```python
from build123d import *

# Parameters (mm, degrees)
ESQUISSE_CYLINDRE_R = 4.5
CYLINDRE_DEPTH      = 29
EPAULEMENT_DEPTH    = 1.5
ESQUISSE_TROU_R     = 2
TROU_DEPTH          = 3.5
CHANFREIN1_SIZE     = 1


with BuildPart() as part:
    # Esquisse_cylindre → Cylindre (new body)
    with BuildSketch(Plane.XY):
        Circle(ESQUISSE_CYLINDRE_R)
    extrude(amount=-CYLINDRE_DEPTH)

    # Esquisse_épaulement → Epaulement (add)
    with BuildSketch(Plane.XY):
        with BuildLine():
            Line((5, 3.31662479), (5, -3.31662479))
            ThreePointArc((5, -3.31662479), (-6, 0), (5, 3.31662479))
        make_face()
    extrude(amount=EPAULEMENT_DEPTH)

    # Esquisse_trou → Trou (cut)
    with BuildSketch(Plane(origin=(0, 0, -29), x_dir=(-1, 0, 0), z_dir=(0, 0, -1))):
        Circle(ESQUISSE_TROU_R)
    extrude(amount=-TROU_DEPTH, mode=Mode.SUBTRACT)

    # Chanfrein1
    chanfrein1_edges = [part.edges().sort_by_distance(p)[0] for p in [
        (-4.5, 0, -29),
    ]]
    chamfer(chanfrein1_edges, length=CHANFREIN1_SIZE)


solid = part.part
```
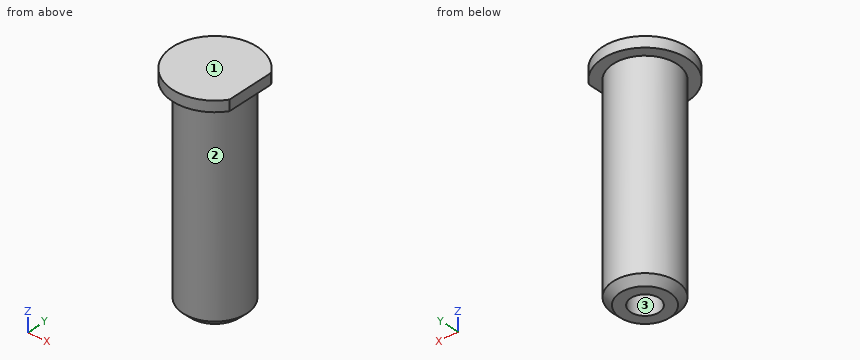
Can you work these out from the model? Positions are in its coordinate system, mm. Face numbers are marked on the shaded views. Coordinates: 2 decimals unless noted, no trailing zeros. Write each loop counter-clockwise with the first axis right and the second up, starting at its lowest first coordinate (ties: lowest second). Pieces come first, ordered by that corner, then holes. Notation, with made-up numbers: (42, 76.25) - (91, 76.25) arc R28 ccw to (91, 99.25) - close; hole circle Ø1 at (-21, 28). An arc over 180 degrees is marked (long way). Return JSON: item names as keys, results as strings.
Q1. If we section it at A-A (y = 0): Please give me the cut outline in (x, z).
Computed values:
{"outline": "(-6, 0) - (-4.5, 0) - (-4.5, -28) - (-3.5, -29) - (-2, -29) - (-2, -25.5) - (2, -25.5) - (2, -29) - (3.5, -29) - (4.5, -28) - (4.5, 0) - (5, 0) - (5, 1.5) - (-6, 1.5) - close"}
Q2. Thinking about a two-plate mould opening in Y: for the marked faces 1, 2 and 3, which applies, +Y half, -Y half, draft (parallel to the pull), parting line (faces both ways), or undercut?
Computed values:
{"face 1": "draft", "face 2": "parting line", "face 3": "undercut"}
Q3. If we section it at C-C (z = -9.5): Please give me the cut outline in (x, y).
Computed values:
{"outline": "circle Ø9 at (0, 0)"}
Q4. If we section it at B-B (x = 0): Please give me the cut outline in (y, z).
Computed values:
{"outline": "(-6, 0) - (-4.5, 0) - (-4.5, -28) - (-3.5, -29) - (-2, -29) - (-2, -25.5) - (2, -25.5) - (2, -29) - (3.5, -29) - (4.5, -28) - (4.5, 0) - (6, 0) - (6, 1.5) - (-6, 1.5) - close"}
Q5. Please list where these lines run through material, in increasing order: L1, parallel to Y at x = 0, z = -26.7; L2, parallel to Z at x = 1.5, y = 5; L3, parallel to Y at x = 1.75, z = -5. Write a range as from..to.
Computed values:
{"L1": "y = -4.5..-2, 2..4.5", "L2": "z = 0..1.5", "L3": "y = -4.15..4.15"}
Q6. I'm going to push flat-ended pins straight in: pin 1 Ø1 at (x, z) = (4, -7) entering from +Y; pin 2 Ø1.5 at (x, z) = (-1, -19.5) entering from +Y; pin 3 Ø1 at (y, z) = (4.5, -14) entering from -X. Where does each tip first touch, or does it pass through?
Computed values:
{"pin 1": "stops at y = 2.83", "pin 2": "stops at y = 4.49", "pin 3": "stops at x = -2.06"}
